Geometry: final body of the model. Coordinates: model frame, mm. Give positions to 0.01 mm unless a question says otherwise; leave off trailing zeros. Loops run counter-clockwise (first coordinate to the right, second up) from the corner with the lowest first, then second, coordinate; pieces in that order, holes last. Notation, with made-up numbers: (44, 37.5) - (54, 37.5) arc R13 ccw to (54, 62.5) - close; hole circle Ø8 at (12, 3). An arc over 180 degrees is marked (long way). Use one line per item in the form item = value.
```python
from build123d import *

# Parameters (mm, degrees)
SKETCH1_W          = 10
SKETCH1_H          = 10
EXTRUDE1_DEPTH     = 170
SKETCH4_R          = 1.5
CUT_EXTRUDE3_DEPTH = 171.587221092
LPATTERN1_COUNT    = 4
LPATTERN1_PITCH    = 50
SKETCH5_R          = 1.5
CUT_EXTRUDE4_DEPTH = 171.587221092


with BuildPart() as part:
    # Sketch1 → Extrude1 (new body)
    with BuildSketch(Plane.XY):
        with Locations((5, 5)):
            Rectangle(SKETCH1_W, SKETCH1_H)
    extrude(amount=EXTRUDE1_DEPTH)

    # Sketch4 → Cut-Extrude3 (cut, through all)
    with BuildSketch(Plane(origin=(0, 10, 0), x_dir=(-1, 0, 0), z_dir=(0, 1, 0))):
        with Locations(Location((-5, 10, 0), (0, 0, 90))):
            Circle(SKETCH4_R)
    cut_extrude3 = extrude(amount=-CUT_EXTRUDE3_DEPTH, mode=Mode.SUBTRACT)

    # LPattern1: Cut-Extrude3 ×4
    with Locations(*[(0, 0, i * LPATTERN1_PITCH) for i in range(1, LPATTERN1_COUNT)]):
        add(cut_extrude3, mode=Mode.SUBTRACT)

    # Sketch5 → Cut-Extrude4 (cut, through all)
    with BuildSketch(Plane.ZY):
        with Locations((20, 5)):
            Circle(SKETCH5_R)
        with Locations((85, 5)):
            Circle(SKETCH5_R)
        with Locations((150, 5)):
            Circle(SKETCH5_R)
    extrude(amount=-CUT_EXTRUDE4_DEPTH, mode=Mode.SUBTRACT)


solid = part.part
```
(1) Pin query (flat end, axial travel): P1, Ø1.8, axis at x = 5, z = 160, coming from the -Y side. Return the tip coordinate at first contact, or that it passes through.
Solution:
P1 = through
(2) Cut plane C-C (y = 5). Return the cut outline in (x, z).
Solution:
outline = (0, 0) - (10, 0) - (10, 18.5) - (0, 18.5) - close; (0, 21.5) - (10, 21.5) - (10, 83.5) - (0, 83.5) - close; (0, 86.5) - (10, 86.5) - (10, 148.5) - (0, 148.5) - close; (0, 151.5) - (10, 151.5) - (10, 170) - (0, 170) - close; hole circle Ø3 at (5, 10); hole circle Ø3 at (5, 60); hole circle Ø3 at (5, 110); hole circle Ø3 at (5, 160)
(3) Material intervals for L1, parallel to Z at x = 5.25, y = 8.75; L2, parallel to Y at x = 5.5, z = 85, sorted ascending. Write a range as from..to.
Solution:
L1 = 0..8.52, 11.48..58.52, 61.48..108.52, 111.48..158.52, 161.48..170
L2 = 0..3.5, 6.5..10
(4) Pull-direction query (X, two-part tool) for faces 1 (the face through (5.07, 5.07, 158.5)), 2 (the face through (5.07, 5.07, 8.5)), 3 (the face through (5, 5, 170)), 4 (the face through (0, 3.8, 83.8)); classes: released by +X, released by -X, zero draft, split by the parting line, or undercut.
Solution:
face_1 = undercut
face_2 = undercut
face_3 = zero draft
face_4 = released by -X
(5) Cut plane B-B (z = 150). Return the cut outline in (x, y).
Solution:
outline = (0, 0) - (10, 0) - (10, 3.5) - (0, 3.5) - close; (0, 6.5) - (10, 6.5) - (10, 10) - (0, 10) - close
(6) Cut plane A-A (x = 5). Return the cut outline in (y, z), plus the area to 3 significant figures.
Solution:
outline = (0, 0) - (10, 0) - (10, 8.5) - (0, 8.5) - close; (0, 11.5) - (10, 11.5) - (10, 58.5) - (0, 58.5) - close; (0, 61.5) - (10, 61.5) - (10, 108.5) - (0, 108.5) - close; (0, 111.5) - (10, 111.5) - (10, 158.5) - (0, 158.5) - close; (0, 161.5) - (10, 161.5) - (10, 170) - (0, 170) - close; hole circle Ø3 at (5, 20); hole circle Ø3 at (5, 85); hole circle Ø3 at (5, 150)
area = 1,560 mm2
